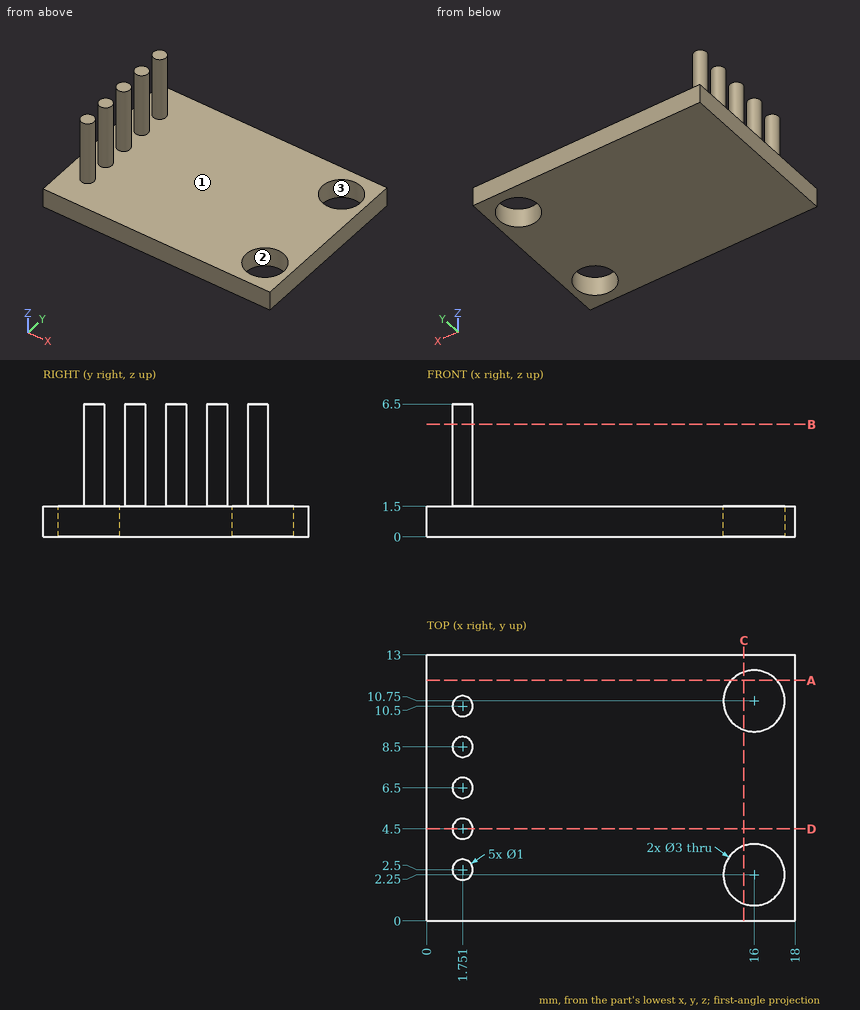
Drawing for the job (mm, zero at the part's lowest x, y, z). Coordinates: 2 decimals unless noted, no trailing zeros. Order: outer loops, then holes, each group sorted by start corner. A loop starts at its lowest first (then second) coordinate and runs counter-clockwise, first axis right, second up. Notation, with made-up numbers: (30, 8.25) -> (35, 8.25) arc R22 ccw to (35, 22.25) -> close; hole circle Ø2 at (18, 57). An arc over 180 degrees is marked (long way). Answer in a Markdown table with one row per item.
1) Band-saw the part on C-C (x = 15.5). List the corners of the cut face in (y, z).
Check values:
| item | result |
|---|---|
| outline | (0, 0) -> (0.84, 0) -> (0.84, 1.5) -> (0, 1.5) -> close; (3.66, 0) -> (9.34, 0) -> (9.34, 1.5) -> (3.66, 1.5) -> close; (12.16, 0) -> (13, 0) -> (13, 1.5) -> (12.16, 1.5) -> close |
2) Band-saw the part on A-A (y = 11.75). List the corners of the cut face in (x, z).
Check values:
| item | result |
|---|---|
| outline | (0, 0) -> (14.88, 0) -> (14.88, 1.5) -> (0, 1.5) -> close; (17.12, 0) -> (18, 0) -> (18, 1.5) -> (17.12, 1.5) -> close |
3) Mould opens along X. For the marked faces 1, 2 and 3 say: pulls with the +X half, pulls with the -X half, needs draft (parallel to the pull), parting line crosses it, or undercut.
Check values:
| item | result |
|---|---|
| face 1 | needs draft |
| face 2 | undercut |
| face 3 | undercut |
4) Band-saw the part on D-D (y = 4.5). List the corners of the cut face in (x, z), and give its area (3 significant figures).
Check values:
| item | result |
|---|---|
| outline | (0, 0) -> (18, 0) -> (18, 1.5) -> (2.25, 1.5) -> (2.25, 6.5) -> (1.25, 6.5) -> (1.25, 1.5) -> (0, 1.5) -> close |
| area | 32.0 mm2 |
5) Flat gauge pins, fed straight in: P1, Ø3.5, axis at x = 16, y = 2.25, coming from the +Z side; P2, Ø2.5, axis at x = 16, y = 10.75, coming from the +Z side; P3, Ø1.5, axis at y = 6, z = 3, coming from the -X side. Where does each tip first touch, or does it go through?
Check values:
| item | result |
|---|---|
| P1 | z = 1.5 |
| P2 | through |
| P3 | x = 1.25 |
6) Band-saw the part on B-B (z = 5.5). List the corners of the cut face in (x, y).
Check values:
| item | result |
|---|---|
| outline | circle Ø1 at (1.75, 2.5); circle Ø1 at (1.75, 4.5); circle Ø1 at (1.75, 6.5); circle Ø1 at (1.75, 8.5); circle Ø1 at (1.75, 10.5) |
7) Drill centre lines: line 1 (Y direction, x = 16, z = 0.8); line 2 (Z direction, x = 4, y = 0.75); line 3 (X direction, y = 8.5, z = 2). Where is each one in solid material? Low to high.
Check values:
| item | result |
|---|---|
| line 1 | 0 to 0.75, 3.75 to 9.25, 12.25 to 13 |
| line 2 | 0 to 1.5 |
| line 3 | 1.25 to 2.25 |
